from build123d import *

# Parameters (mm, degrees)
RESSALTO_EXTRUS_O1_DEPTH = 120
ESBO_O3_R                = 0.675
CORTE_EXTRUS_O1_DEPTH    = 30


with BuildPart() as part:
    # Esboço1 → Ressalto-extrusão1 (new body)
    with BuildSketch(Plane.XY):
        with BuildLine():
            Line((35, -12.5), (35, 22.5))
            Line((35, 22.5), (-35, 22.5))
            Line((-35, 22.5), (-35, -12.5))
            Line((-35, -12.5), (-0.384609579, -22.390111549))
            ThreePointArc((-0.384609579, -22.390111549), (0.017433528, -22.081919349), (0.42886001, -22.377468569))
            Line((0.42886001, -22.377468569), (35, -12.5))
        make_face()
    extrude(amount=RESSALTO_EXTRUS_O1_DEPTH)

    # Esboço3 → Corte-extrusão1 (cut)
    with BuildSketch(Plane.XY.offset(120)):
        with Locations((0, -22.5)):
            Circle(ESBO_O3_R)
    extrude(amount=-CORTE_EXTRUS_O1_DEPTH, mode=Mode.SUBTRACT)


solid = part.part
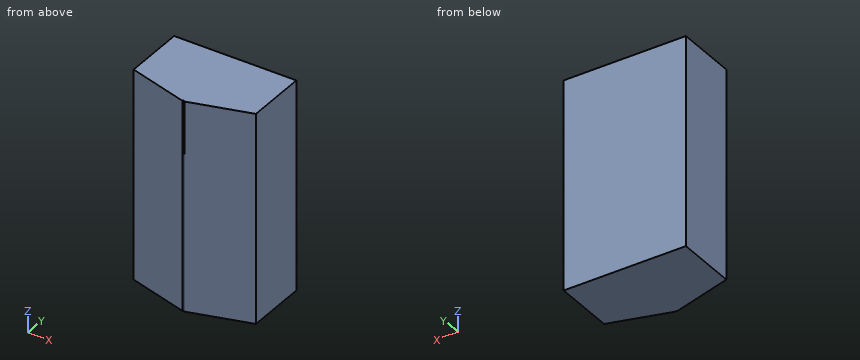
The model under review builds one solid part; all positions refer to its coordinate system, in mm. Round coordinates to 2 decimals unless told otherwise and drop trailing zeros. Loops run counter-clockwise (first coordinate to the right, second up) from the corner with the lowest first, then second, coordinate; pieces in that order, holes last. Notation, with made-up numbers: (45, 40.5) -> (75, 40.5) arc R29 ccw to (75, 69.5) -> close; hole circle Ø9 at (-26.5, 38.5). An arc over 180 degrees is marked (long way). Answer as CSV lines item,"result".
1) For P1, Ø8, axis at x = 17.5, y = 16, coming from the -Z side, flat-tipped, find the tip position at first contact; note if it passes through.
Geometry results:
P1,"stops at z = 0"
2) To check wall thickness, follow line 1 along Y through (x, z) = (-18.5, 106); line 2 along Y through (x, z) = (-26.5, 82). State the ranges of each line that lie inside material, in increasing order. Write a range as from..to.
Geometry results:
line 1,"y = -17.21..22.5"
line 2,"y = -14.93..22.5"
3) Add section C-C on z = 97. Write out the cut boundary in (x, y) (3 decimals), plus the area to 3 significant figures.
Geometry results:
outline,"(-35, -12.5) -> (-0.649, -22.315) arc R0.675 cw to (0.649, -22.315) -> (35, -12.5) -> (35, 22.5) -> (-35, 22.5) -> close"
area,"2,800 mm²"
4) Add section A-A on z = 56.5. Write out the cut boundary in (x, y) (3 decimals).
Geometry results:
outline,"(-35, -12.5) -> (-0.385, -22.39) arc R0.425 cw to (0.429, -22.377) -> (35, -12.5) -> (35, 22.5) -> (-35, 22.5) -> close"
5) Add section B-B on x = -14. Write out the cut boundary in (y, z), plus the area to 3 significant figures.
Geometry results:
outline,"(-18.5, 0) -> (22.5, 0) -> (22.5, 120) -> (-18.5, 120) -> close"
area,"4,920 mm²"
6) Add section D-D on x = 25. Write out the cut boundary in (y, z).
Geometry results:
outline,"(-15.36, 0) -> (22.5, 0) -> (22.5, 120) -> (-15.36, 120) -> close"
